Design review of the part built by this model. Coordinates are the model's own, in mm. A direction names the side the tool comes from. Coordinates: 2 decimals unless noted, no trailing zeros. Order: outer loops, then holes, each group sorted by start corner. A loop starts at its lowest first (then second) coordinate and runs counter-clockwise, first axis right, second up. Notation, with made-up numbers: M 0,-15 L 50,-15 A34 cw 50,23 Z; hole C -35.75,5 d11. An arc over 180 degrees is marked long. Answer in a Markdown table with one row per item.
from build123d import *

# Parameters (mm, degrees)
SKETCH_1_R          = 60
EXTRUDE_1_DEPTH     = 50
SKETCH_2_R          = 3
CUT_EXTRUDE_1_DEPTH = 10
SHELL_START         = -50
SHELL_1_DEPTH       = 45
SHELL_1_2_DEPTH     = 35
SKETCH_3_W          = 45
SKETCH_3_H          = 45
SKETCH_3_W_2        = 43.3
SKETCH_3_H_2        = 43.3
EXTRUDE_2_DEPTH     = 25
SKETCH_4_R          = 5
CUT_EXTRUDE_2_DEPTH = 97.046863561
SKETCH_5_W          = 30
SKETCH_5_H          = 20
SKETCH_5_W_2        = 20
SKETCH_5_H_2        = 30
CUT_EXTRUDE_3_DEPTH = 20
SKETCH_6_W          = 24.083269132
SKETCH_6_H          = 5
SKETCH_6_W_2        = 5
SKETCH_6_H_2        = 24.083269132
EXTRUDE_3_DEPTH     = 20
SKETCH_7_R          = 3
EXTRUDE_4_DEPTH     = 20
EXTRUDE_5_REACH     = 106.881
SKETCH_8_R          = 3
SKETCH_10_R         = 2.5
EXTRUDE_6_DEPTH     = 10
SKETCH_11_W         = 100
SKETCH_11_H         = 100
CUT_EXTRUDE_4_DEPTH = 40


# Read off the part's stored shape, not the designer's step: 抽壳1
with BuildPart() as part:
    # 草图1 → 凸台-拉伸1 (new body)
    with BuildSketch(Plane.XY):
        Circle(SKETCH_1_R)
    extrude(amount=-EXTRUDE_1_DEPTH)

    # 草图2 → 切除-拉伸1 (cut)
    with BuildSketch(Plane.XY):
        with Locations((34, 34)):
            Circle(SKETCH_2_R)
        with Locations((34, -34)):
            Circle(SKETCH_2_R)
        with Locations((-34, -34)):
            Circle(SKETCH_2_R)
        with Locations((-34, 34)):
            Circle(SKETCH_2_R)
    extrude(amount=-CUT_EXTRUDE_1_DEPTH, mode=Mode.SUBTRACT)

    # 抽壳1 outline → 抽壳1 (cut)
    with BuildSketch(Plane.XY.offset(SHELL_START)):
        with BuildLine():
            ThreePointArc((41.809731384, -35.734386263), (55, 0), (41.809731384, 35.734386263))
            ThreePointArc((41.809731384, 35.734386263), (28.343145751, 28.343145751), (35.734386263, 41.809731384))
            ThreePointArc((35.734386263, 41.809731384), (0, 55), (-35.734386263, 41.809731384))
            ThreePointArc((-35.734386263, 41.809731384), (-28.343145751, 28.343145751), (-41.809731384, 35.734386263))
            ThreePointArc((-41.809731384, 35.734386263), (-55, 0), (-41.809731384, -35.734386263))
            ThreePointArc((-41.809731384, -35.734386263), (-28.343145751, -28.343145751), (-35.734386263, -41.809731384))
            ThreePointArc((-35.734386263, -41.809731384), (0, -55), (35.734386263, -41.809731384))
            ThreePointArc((35.734386263, -41.809731384), (28.343145751, -28.343145751), (41.809731384, -35.734386263))
        make_face()
    extrude(amount=SHELL_1_DEPTH, mode=Mode.SUBTRACT)

    # Shell 1 2 outline → Shell 1 2 (cut)
    with BuildSketch(Plane.XY.offset(SHELL_START)):
        with BuildLine():
            ThreePointArc((35.734386263, 41.809731384), (28.343145751, 28.343145751), (41.809731384, 35.734386263))
            ThreePointArc((41.809731384, 35.734386263), (38.890872965, 38.890872965), (35.734386263, 41.809731384))
        make_face()
        with BuildLine():
            ThreePointArc((35.734386263, -41.809731384), (38.890872965, -38.890872965), (41.809731384, -35.734386263))
            ThreePointArc((41.809731384, -35.734386263), (28.343145751, -28.343145751), (35.734386263, -41.809731384))
        make_face()
        with BuildLine():
            ThreePointArc((-41.809731384, 35.734386263), (-28.343145751, 28.343145751), (-35.734386263, 41.809731384))
            ThreePointArc((-35.734386263, 41.809731384), (-38.890872965, 38.890872965), (-41.809731384, 35.734386263))
        make_face()
        with BuildLine():
            ThreePointArc((-41.809731384, -35.734386263), (-38.890872965, -38.890872965), (-35.734386263, -41.809731384))
            ThreePointArc((-35.734386263, -41.809731384), (-28.343145751, -28.343145751), (-41.809731384, -35.734386263))
        make_face()
    extrude(amount=SHELL_1_2_DEPTH, mode=Mode.SUBTRACT)

    # 草图3 → 凸台-拉伸2 (add)
    with BuildSketch(Plane.XY):
        Rectangle(SKETCH_3_W, SKETCH_3_H)
        Rectangle(SKETCH_3_W_2, SKETCH_3_H_2, mode=Mode.SUBTRACT)
    extrude(amount=-EXTRUDE_2_DEPTH)

    # 草图4 → 切除-拉伸2 (cut, through all)
    with BuildSketch(Plane(origin=(0, 0, -5), x_dir=(-1, 0, 0), z_dir=(0, 0, -1))):
        Circle(SKETCH_4_R)
    extrude(amount=-CUT_EXTRUDE_2_DEPTH, mode=Mode.SUBTRACT)

    # 草图5 → 切除-拉伸3 (cut)
    with BuildSketch(Plane.XY):
        with Locations((-45, 0)):
            Rectangle(SKETCH_5_W, SKETCH_5_H)
        with Locations((0, 45)):
            Rectangle(SKETCH_5_W_2, SKETCH_5_H_2)
        with Locations((45, 0)):
            Rectangle(SKETCH_5_W, SKETCH_5_H)
        with Locations((0, -45)):
            Rectangle(SKETCH_5_W_2, SKETCH_5_H_2)
    extrude(amount=-CUT_EXTRUDE_3_DEPTH, mode=Mode.SUBTRACT)

    # 草图6 → 凸台-拉伸3 (add)
    with BuildSketch(Plane(origin=(0, 0, -5), x_dir=(-1, 0, 0), z_dir=(0, 0, -1))):
        with Locations((-42.041634566, 12.5)):
            Rectangle(SKETCH_6_W, SKETCH_6_H)
        with Locations((-42.041634566, -12.5)):
            Rectangle(SKETCH_6_W, SKETCH_6_H)
        with Locations((12.5, 42.041634566)):
            Rectangle(SKETCH_6_W_2, SKETCH_6_H_2)
        with Locations((-12.5, 42.041634566)):
            Rectangle(SKETCH_6_W_2, SKETCH_6_H_2)
        with Locations((42.041634566, -12.5)):
            Rectangle(SKETCH_6_W, SKETCH_6_H)
        with Locations((42.041634566, 12.5)):
            Rectangle(SKETCH_6_W, SKETCH_6_H)
        with Locations((-12.5, -42.041634566)):
            Rectangle(SKETCH_6_W_2, SKETCH_6_H_2)
        with Locations((12.5, -42.041634566)):
            Rectangle(SKETCH_6_W_2, SKETCH_6_H_2)
    extrude(amount=EXTRUDE_3_DEPTH)

    # 草图7 → 凸台-拉伸4 (add)
    with BuildSketch(Plane.ZY.offset(-10)):
        with Locations(Location((-10, 55, 0), (0, 0, 180))):
            Circle(SKETCH_7_R)
        with Locations(Location((-10, -55, 0), (0, 0, 90))):
            Circle(SKETCH_7_R)
    extrude(amount=EXTRUDE_4_DEPTH)

    # 草图8 → 凸台-拉伸5 (add, up to next)
    with BuildSketch(Plane.XZ.offset(-10), mode=Mode.PRIVATE) as extrude_5_sk1:
        with Locations(Location((55, -10, 0), (0, 0, 180))):
            Circle(SKETCH_8_R)
    extrude_5_tool1 = extrude(extrude_5_sk1.sketch, amount=EXTRUDE_5_REACH, mode=Mode.PRIVATE) - part.part
    # 草图8 → 凸台-拉伸5 (add, up to next)
    with BuildSketch(Plane.XZ.offset(-10), mode=Mode.PRIVATE) as extrude_5_sk2:
        with Locations(Location((-55, -10, 0), (0, 0, 90))):
            Circle(SKETCH_8_R)
    extrude_5_tool2 = extrude(extrude_5_sk2.sketch, amount=EXTRUDE_5_REACH, mode=Mode.PRIVATE) - part.part
    add(extrude_5_tool1.solids().sort_by_distance((55, 10, -10))[0])
    add(extrude_5_tool2.solids().sort_by_distance((-55, 10, -10))[0])

    # 草图10 → 凸台-拉伸6 (add)
    # profile 1 of 4: a face of its own
    with BuildSketch(Plane.XY):
        with BuildLine():
            Line((-48.904069139, 34.761933515), (-52.68935793, 42.789862994))
            ThreePointArc((-52.68935793, 42.789862994), (-51.221228705, 51.221228705), (-42.789862994, 52.68935793))
            Line((-42.789862994, 52.68935793), (-34.761933515, 48.904069139))
            ThreePointArc((-34.761933515, 48.904069139), (-42.426406871, 42.426406871), (-48.904069139, 34.761933515))
        make_face()
        with Locations((-45, 45)):
            Circle(SKETCH_10_R, mode=Mode.SUBTRACT)
    # profile 2 of 4: a face of its own
    with BuildSketch(Plane.XY):
        with BuildLine():
            Line((34.761933515, 48.904069139), (42.789862994, 52.68935793))
            ThreePointArc((42.789862994, 52.68935793), (51.221228705, 51.221228705), (52.68935793, 42.789862994))
            Line((52.68935793, 42.789862994), (48.904069139, 34.761933515))
            ThreePointArc((48.904069139, 34.761933515), (42.426406871, 42.426406871), (34.761933515, 48.904069139))
        make_face()
        with Locations(Location((45, 45, 0), (0, 0, 180))):
            Circle(SKETCH_10_R, mode=Mode.SUBTRACT)
    # profile 3 of 4: a face of its own
    with BuildSketch(Plane.XY):
        with BuildLine():
            Line((48.904069139, -34.761933515), (52.68935793, -42.789862994))
            ThreePointArc((52.68935793, -42.789862994), (51.221228705, -51.221228705), (42.789862994, -52.68935793))
            Line((42.789862994, -52.68935793), (34.761933515, -48.904069139))
            ThreePointArc((34.761933515, -48.904069139), (42.426406871, -42.426406871), (48.904069139, -34.761933515))
        make_face()
        with Locations((45, -45)):
            Circle(SKETCH_10_R, mode=Mode.SUBTRACT)
    # profile 4 of 4: a face of its own
    with BuildSketch(Plane.XY):
        with BuildLine():
            Line((-34.761933515, -48.904069139), (-42.789862994, -52.68935793))
            ThreePointArc((-42.789862994, -52.68935793), (-51.221228705, -51.221228705), (-52.68935793, -42.789862994))
            Line((-52.68935793, -42.789862994), (-48.904069139, -34.761933515))
            ThreePointArc((-48.904069139, -34.761933515), (-42.426406871, -42.426406871), (-34.761933515, -48.904069139))
        make_face()
        with Locations(Location((-45, -45, 0), (0, 0, 180))):
            Circle(SKETCH_10_R, mode=Mode.SUBTRACT)
    extrude(amount=-EXTRUDE_6_DEPTH)

    # 草图11 → 切除-拉伸4 (cut)
    with BuildSketch(Plane(origin=(0, 0, -50), x_dir=(-1, 0, 0), z_dir=(0, 0, -1))):
        Rectangle(SKETCH_11_W, SKETCH_11_H)
    extrude(amount=-CUT_EXTRUDE_4_DEPTH, mode=Mode.SUBTRACT)


solid = part.part
(1) Draft analysis for pull direction Y (two halves, no side actions). For faces 5 (the flat face through (-12, -50, -18)), 6 (the flat face through (-38.832, 50.823, -4.93)), 7 (the flat face through (-50, -28, -30)), state which applies: pulls with the +Y half, pulls with the -Y half, needs draft (parallel to the pull), parting line crosses it, or undercut.
Return value:
| item | result |
|---|---|
| face 5 | undercut |
| face 6 | pulls with the +Y half |
| face 7 | needs draft |
(2) For faces 1 (the flat face through (50.77, -38.72, -4.93)), 2 (the flat face through (-12, 50, -18)), 3 (the flat face through (-30, 0, -2)), 4 (the flat face through (22.5, 0, -7)), list the 3-axis set-ups (+Z, -Z, +X, -X, +Y, -Y) from which the entire face can be reached by the end or side of a thin tool; tool diameter is ignored.
Return value:
| item | result |
|---|---|
| face 1 | +Z, -Z, +X |
| face 2 | -Z, +X, -X |
| face 3 | +Z, -Z, -X |
| face 4 | -Z |
(3) Add section B-B, the plane z = -26.5. Give the boundary of the cut face in (x, y).
Return value:
| item | result |
|---|---|
| outline | M -50,-33.17 L -50,-22.91 A55 cw -50,22.91 L -50,33.17 A60 ccw Z; M -33.17,-50 A60 ccw 33.17,-50 L 22.91,-50 A55 cw -22.91,-50 Z; M -33.17,50 L -22.91,50 A55 cw 22.91,50 L 33.17,50 A60 ccw Z; M 50,-33.17 A60 ccw 50,33.17 L 50,22.91 A55 cw 50,-22.91 Z |
(4) Add section C-C, the plane x = -45. Give the boundary of the cut face in (y, z).
Return value:
| item | result |
|---|---|
| outline | M -53.34,-10 L -47.5,-10 L -47.5,0 L -53.34,0 Z; M -42.5,-10 L -31.62,-10 L -31.62,-5 L -15,-5 L -15,-10 L -10,-10 L -10,0 L -42.5,0 Z; M 10,-10 L 15,-10 L 15,-5 L 31.62,-5 L 31.62,-10 L 42.5,-10 L 42.5,0 L 10,0 Z; M 47.5,-10 L 53.34,-10 L 53.34,0 L 47.5,0 Z |
(5) Insertion check: pin 1 Ø3 at (x, z) = (30, -35) entering from -Y; pin 2 Ø20 at (x, z) = (-51, -7) entering from -Y; pin 3 Ø6 at (y, z) = (-9.5, -43) entering from -X. Each pin has a flat end and moves straight along its axis. Give the tip position at first contact, or say it passes through.
Return value:
| item | result |
|---|---|
| pin 1 | stops at y = -52.8 |
| pin 2 | stops at y = -53.4 |
| pin 3 | stops at x = -59.65 |
(6) For line 1 along Y through (x, z) = (45, -6); line 2 along Y through (x, z) = (0, -3.5); line 3 along Z through (x, y) = (-52, 11), list the stretches that pass through material, from the lowest coordinate up. Write a range as from..to.
Return value:
| item | result |
|---|---|
| line 1 | y = -53.34..-47.5, -42.5..-31.62, -15..-10, 10..15, 31.62..42.5, 47.5..53.34 |
| line 2 | y = -30..-5, 5..30 |
| line 3 | z = -25..0 |
(7) Add section A-A, the plane y = 0. Give the boundary of the cut face in (x, z), and give its area (3 significant figures).
Return value:
| item | result |
|---|---|
| outline | M -60,-50 L -55,-50 L -55,-20 L -60,-20 Z; C -55,-10 d6; M -30,-5 L -22.5,-5 L -22.5,-10 L -21.65,-10 L -21.65,-5 L -5,-5 L -5,0 L -30,0 Z; M 5,-5 L 21.65,-5 L 21.65,-10 L 22.5,-10 L 22.5,-5 L 30,-5 L 30,0 L 5,0 Z; C 55,-10 d6; M 55,-50 L 60,-50 L 60,-20 L 55,-20 Z |
| area | 615 mm2 |
